Check sheet for the modelled part. Datum: model origin and axes. Units: mm. Coordinates: 2 decimals unless noted, no trailing zeros. Loops run counter-clockwise (first coordinate to the right, second up) from the corner with the lowest first, then second, coordinate; pieces in that order, holes last.
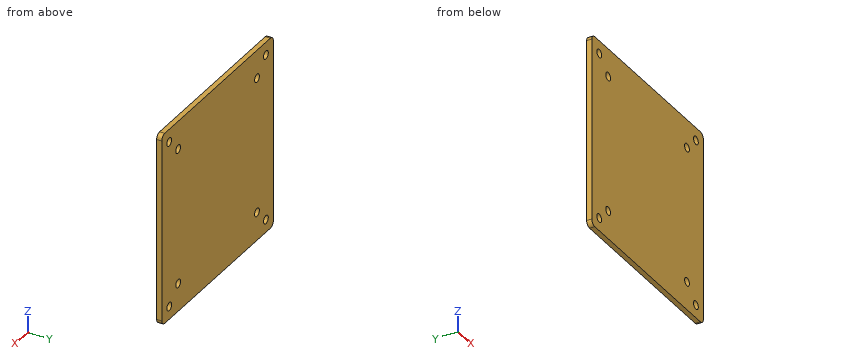
```python
from build123d import *

# Parameters (mm, degrees)
SKETCH_1_W      = 75
SKETCH_1_H      = 75
SKETCH_1_R      = 1.6
EXTRUDE_1_DEPTH = 2
FILLET_1_R      = 2


with BuildPart() as part:
    # 草图1 → 凸台-拉伸1 (new body)
    with BuildSketch(Plane(origin=(0, 0, 0), x_dir=(1, 0, 0), z_dir=(0, 1, 0))):
        Rectangle(SKETCH_1_W, SKETCH_1_H)
        with Locations(Location((-26.5, 26.5, 0), (0, 0, 270))):
            Circle(SKETCH_1_R, mode=Mode.SUBTRACT)
        with Locations(Location((26.5, 26.5, 0), (0, 0, 270))):
            Circle(SKETCH_1_R, mode=Mode.SUBTRACT)
        with Locations(Location((26.5, -26.5, 0), (0, 0, 90))):
            Circle(SKETCH_1_R, mode=Mode.SUBTRACT)
        with Locations(Location((-26.5, -26.5, 0), (0, 0, 90))):
            Circle(SKETCH_1_R, mode=Mode.SUBTRACT)
        with Locations(Location((-32.5, 32.5, 0), (0, 0, 270))):
            Circle(SKETCH_1_R, mode=Mode.SUBTRACT)
        with Locations(Location((32.5, 32.5, 0), (0, 0, 270))):
            Circle(SKETCH_1_R, mode=Mode.SUBTRACT)
        with Locations(Location((32.5, -32.5, 0), (0, 0, 90))):
            Circle(SKETCH_1_R, mode=Mode.SUBTRACT)
        with Locations(Location((-32.5, -32.5, 0), (0, 0, 90))):
            Circle(SKETCH_1_R, mode=Mode.SUBTRACT)
    extrude(amount=EXTRUDE_1_DEPTH)

    # 圆角1
    fillet_1_edges = [part.edges().sort_by_distance(p)[0] for p in [
        (37.5, 1, 37.5),
        (-37.5, 1, 37.5),
        (-37.5, 1, -37.5),
        (37.5, 1, -37.5),
    ]]
    fillet(fillet_1_edges, radius=FILLET_1_R)


solid = part.part
```
1) Scan lines: line 1 (X direction, y = 1.15, z = 26.5); line 2 (X direction, y = 1.55, z = 32.5); line 3 (Z direction, x = 26, y = 0.15). Record each from-to range of solid material in increasing order.
Answer sheet:
line 1: x = -37.5 to -28.1, -24.9 to 24.9, 28.1 to 37.5
line 2: x = -37.5 to -34.1, -30.9 to 30.9, 34.1 to 37.5
line 3: z = -37.5 to -28.02, -24.98 to 24.98, 28.02 to 37.5
2) Section check A-A on z = -26.5. Enter the section's corners in (x, y), plus the area to 3 significant figures.
Answer sheet:
outline: (-37.5, 0) - (-28.1, 0) - (-28.1, 2) - (-37.5, 2) - close; (-24.9, 0) - (24.9, 0) - (24.9, 2) - (-24.9, 2) - close; (28.1, 0) - (37.5, 0) - (37.5, 2) - (28.1, 2) - close
area: 137 mm2
3) Section check B-B on x = 32.5. Enter the section's corners in (y, z).
Answer sheet:
outline: (0, -37.5) - (2, -37.5) - (2, -34.1) - (0, -34.1) - close; (0, -30.9) - (2, -30.9) - (2, 30.9) - (0, 30.9) - close; (0, 34.1) - (2, 34.1) - (2, 37.5) - (0, 37.5) - close
4) Depth check by flat-ended pin: pin 1 (1.9 mm diameter, centred on x = -32.5, z = -32.5, fed in from +Y); pin 2 (5 mm diameter, centred on x = 26.5, z = -26.5, fed in from -Y). Enter the tip coordinate at first touch or a pass-through.
Answer sheet:
pin 1: passes through
pin 2: stops at y = 0
